Design review of the part built by this model. Coordinates are the model's own, in mm. A direction names the side the tool comes from. Round coordinates to 2 decimals unless told otherwise and drop trailing zeros. Write each loop counter-clockwise with the first axis right and the second up, starting at its lowest first coordinate (ties: lowest second). Pieces come first, ordered by that corner, then holes. Notation, with made-up numbers: M 67.25,-34 L 98.25,-34 A32 ccw 98.25,-8 Z; hole C 16.25,8.5 d11. An arc over 180 degrees is marked long. Use CSV: the item, a comma, the result in double quotes.
from build123d import *

# Parameters (mm, degrees)
F0_R     = 150
F0_R_2   = 3.75
F0_R_3   = 2.1
F1_DEPTH = 10
F2_DEPTH = 4.2


with BuildPart() as f1:
    # F0 (on Top) → F1 (new body)
    with BuildSketch(Plane.XY):
        Circle(F0_R)
        with Locations((-122.975607, -71)):
            Circle(F0_R_2, mode=Mode.SUBTRACT)
        with Locations((122.975607, -71)):
            Circle(F0_R_2, mode=Mode.SUBTRACT)
        with Locations((0, 142)):
            Circle(F0_R_2, mode=Mode.SUBTRACT)
        with Locations((0, 142)):
            Circle(F0_R_2)
        with Locations((0, 142)):
            Circle(F0_R_3, mode=Mode.SUBTRACT)
        with Locations((122.975607, -71)):
            Circle(F0_R_2)
        with Locations((122.975607, -71)):
            Circle(F0_R_3, mode=Mode.SUBTRACT)
        with Locations((-122.975607, -71)):
            Circle(F0_R_2)
        with Locations((-122.975607, -71)):
            Circle(F0_R_3, mode=Mode.SUBTRACT)
    extrude(amount=F1_DEPTH)

    # F0 (on Top) → F2 (cut)
    with BuildSketch(Plane.XY):
        with Locations((-122.975607, -71)):
            Circle(F0_R_2)
        with Locations((-122.975607, -71)):
            Circle(F0_R_3, mode=Mode.SUBTRACT)
        with Locations((122.975607, -71)):
            Circle(F0_R_2)
        with Locations((122.975607, -71)):
            Circle(F0_R_3, mode=Mode.SUBTRACT)
        with Locations((0, 142)):
            Circle(F0_R_2)
        with Locations((0, 142)):
            Circle(F0_R_3, mode=Mode.SUBTRACT)
    extrude(amount=F2_DEPTH, mode=Mode.SUBTRACT)


solid = f1.part
1) Machinability: for faces 5 (the face through (-2, 2, 0)), 6 (the face through (-121, -73, 4.2)), which of the approach directions +Z, -Z, +X, -X, +Y, -Y give a long, thin tool a straight path to every point of the face, cutting with its end or side? Answer none if there is none.
Answers:
face 5,"-Z, +X, -X, +Y, -Y"
face 6,"-Z"
2) Add section A-A on z = 8.25. Write out the cut boundary in (x, y).
Answers:
outline,"C 0,0 d300; hole C -122.98,-71 d4.2; hole C 0,142 d4.2; hole C 122.98,-71 d4.2"
3) Add section C-C on x = 46. Write out the cut boundary in (y, z).
Answers:
outline,"M -142.77,0 L 142.77,0 L 142.77,10 L -142.77,10 Z"
4) For pin 1 Ø1.5 at (y, z) = (-62, 5) entering from -X; pin 2 Ø6.5 at (x, y) = (-122.98, -71) entering from -Z; pin 3 Ø3 at (x, z) = (-116, 6) entering from +Y, all flat-tipped, find the tip position at first contact; note any pin that passes through.
Answers:
pin 1,"x = -136.92"
pin 2,"z = 4.2"
pin 3,"y = 96.9"
5) Wall thickness on line 1 along Y through (x, z) = (0, 2.65); line 2 along Y through (x, z) = (0, 6.35); line 3 along Y through (x, z) = (25, 5): over which ranges is each line inside the solid? List them lowest first. Write a range as [from, to].
Answers:
line 1,"[-150, 138.25], [145.75, 150]"
line 2,"[-150, 139.9], [144.1, 150]"
line 3,"[-147.9, 147.9]"
6) The part is to be moulded in two halves that separate along Y. For faces 1 (the face through (-19.527, 148.724, 4.93)), 2 (the face through (-2, 2, 10)), 3 (the face through (120.21, -68.47, 2.07)), 4 (the face through (125, -73, 4.2)), say which applies: released by +Y, released by -Y, zero draft, split by the parting line, or undercut.
Answers:
face 1,"split by the parting line"
face 2,"zero draft"
face 3,"undercut"
face 4,"undercut"
7) Add section B-B on y = -122.5. Write out the cut boundary in (x, z).
Answers:
outline,"M -86.57,0 L 86.57,0 L 86.57,10 L -86.57,10 Z"
